Read the model definition and answer for the solid it produces. Units are mm, in the model's axes. A direction names the side the tool comes from. Coordinates: 2 decimals unless noted, no trailing zeros. Order: outer loops, then holes, each group sorted by start corner. A loop starts at its lowest first (then second) coordinate and runs counter-clockwise, first axis right, second up. Notation, with made-up numbers: (-27, -20) -> (2, -20) arc R20 cw to (2, -13) -> close; hole circle Ø10 at (40.25, 68). An arc over 180 degrees is marked (long way). Use CSV: the item, a comma, the result in double quotes.
```python
from build123d import *

# Parameters (mm, degrees)
BOSS_EXTRUDE1_DEPTH = 20.9804
CUT_EXTRUDE1_DEPTH  = 15.9004


with BuildPart() as part:
    # Sketch1 → Boss-Extrude1 (new body)
    with BuildSketch(Plane(origin=(0, 0, 0), x_dir=(1, 0, 0), z_dir=(0, 1, 0))):
        with BuildLine():
            Line((0, -8.255), (0, -23.876))
            ThreePointArc((0, -23.876), (0.92993597, -26.12106403), (3.175, -27.051))
            Line((3.175, -27.051), (16.330087154, -27.051))
            ThreePointArc((16.330087154, -27.051), (18.092140644, -27.584827438), (19.261669723, -29.0068))
            ThreePointArc((19.261669723, -29.0068), (30.988, -36.83), (42.714330277, -29.0068))
            ThreePointArc((42.714330277, -29.0068), (43.883859356, -27.584827438), (45.645912846, -27.051))
            Line((45.645912846, -27.051), (58.801, -27.051))
            ThreePointArc((58.801, -27.051), (61.04606403, -26.12106403), (61.976, -23.876))
            Line((61.976, -23.876), (61.976, -8.255))
            ThreePointArc((61.976, -8.255), (58.256256121, 0.725256121), (49.276, 4.445))
            Line((49.276, 4.445), (12.7, 4.445))
            ThreePointArc((12.7, 4.445), (3.719743879, 0.725256121), (0, -8.255))
        make_face()
        with BuildLine():
            Line((13.208, -10.541), (22.733, -10.541))
            ThreePointArc((22.733, -10.541), (25.908, -13.716), (22.733, -16.891))
            Line((22.733, -16.891), (13.208, -16.891))
            ThreePointArc((13.208, -16.891), (10.033, -13.716), (13.208, -10.541))
        make_face(mode=Mode.SUBTRACT)
        with BuildLine():
            Line((48.768, -10.541), (39.243, -10.541))
            ThreePointArc((39.243, -10.541), (36.068, -13.716), (39.243, -16.891))
            Line((39.243, -16.891), (48.768, -16.891))
            ThreePointArc((48.768, -16.891), (51.943, -13.716), (48.768, -10.541))
        make_face(mode=Mode.SUBTRACT)
    extrude(amount=BOSS_EXTRUDE1_DEPTH)

    # Sketch2 → Cut-Extrude1 (cut)
    with BuildSketch(Plane(origin=(0, 20.9804, 0), x_dir=(1, 0, 0), z_dir=(0, 1, 0))):
        with BuildLine():
            Line((6.858, -9.525), (6.858, -17.907))
            ThreePointArc((6.858, -17.907), (7.78793597, -20.15206403), (10.033, -21.082))
            Line((10.033, -21.082), (25.908, -21.082))
            ThreePointArc((25.908, -21.082), (28.15306403, -20.15206403), (29.083, -17.907))
            Line((29.083, -17.907), (29.083, -9.525))
            ThreePointArc((29.083, -9.525), (28.15306403, -7.27993597), (25.908, -6.35))
            Line((25.908, -6.35), (10.033, -6.35))
            ThreePointArc((10.033, -6.35), (7.78793597, -7.27993597), (6.858, -9.525))
        make_face()
        with BuildLine():
            Line((51.943, -6.35), (36.068, -6.35))
            ThreePointArc((36.068, -6.35), (33.82293597, -7.27993597), (32.893, -9.525))
            Line((32.893, -9.525), (32.893, -17.907))
            ThreePointArc((32.893, -17.907), (33.82293597, -20.15206403), (36.068, -21.082))
            Line((36.068, -21.082), (51.943, -21.082))
            ThreePointArc((51.943, -21.082), (54.18806403, -20.15206403), (55.118, -17.907))
            Line((55.118, -17.907), (55.118, -9.525))
            ThreePointArc((55.118, -9.525), (54.18806403, -7.27993597), (51.943, -6.35))
        make_face()
    extrude(amount=-CUT_EXTRUDE1_DEPTH, mode=Mode.SUBTRACT)


solid = part.part
```
Item 1: A tool of negligible diameter and unlimited length cuts with its end or side. For faces 1 (the cylindrical face through (33.8, 13.14, 20.13)), 2 (the flat face through (44, 3, 10.541)), 3 (the flat face through (52, 10, 27.051)), from which of +Z, -Z, +X, -X, +Y, -Y can it reach the whole face along a straight path? Write none if from no direction.
Return value:
face 1,"+Y"
face 2,"+Y, -Y"
face 3,"+Z, +X, +Y, -Y"
Item 2: Find section D-D, the plane y = 4. Give the vertices of the cut face in (x, z) (3 decimals), then the cut area to 3 significant figures.
Return value:
outline,"(0, 8.255) arc R12.7 ccw to (12.7, -4.445) -> (49.276, -4.445) arc R12.7 ccw to (61.976, 8.255) -> (61.976, 23.876) arc R3.175 ccw to (58.801, 27.051) -> (45.646, 27.051) arc R3.175 cw to (42.714, 29.007) arc R12.7 ccw to (19.262, 29.007) arc R3.175 cw to (16.33, 27.051) -> (3.175, 27.051) arc R3.175 ccw to (0, 23.876) -> close; hole (13.208, 10.541) -> (22.733, 10.541) arc R3.175 ccw to (22.733, 16.891) -> (13.208, 16.891) arc R3.175 ccw to start; hole (39.243, 10.541) -> (48.768, 10.541) arc R3.175 ccw to (48.768, 16.891) -> (39.243, 16.891) arc R3.175 ccw to start"
area,"1,880 mm^2"
Item 3: Find section B-B, the plane z = 15. Give the vertices of the cut face in (x, y), then the cut area to 3 significant figures.
Return value:
outline,"(0, 0) -> (10.3, 0) -> (10.3, 5.08) -> (6.86, 5.08) -> (6.86, 20.98) -> (0, 20.98) -> close; (25.64, 0) -> (36.34, 0) -> (36.34, 5.08) -> (32.89, 5.08) -> (32.89, 20.98) -> (29.08, 20.98) -> (29.08, 5.08) -> (25.64, 5.08) -> close; (51.67, 0) -> (61.98, 0) -> (61.98, 20.98) -> (55.12, 20.98) -> (55.12, 5.08) -> (51.67, 5.08) -> close"
area,"438 mm^2"
Item 4: Find section A-A, the plane y = 7.5. Give the vertices of the cut face in (x, z) (3 decimals), then the cut area to 3 significant figures.
Return value:
outline,"(0, 8.255) arc R12.7 ccw to (12.7, -4.445) -> (49.276, -4.445) arc R12.7 ccw to (61.976, 8.255) -> (61.976, 23.876) arc R3.175 ccw to (58.801, 27.051) -> (45.646, 27.051) arc R3.175 cw to (42.714, 29.007) arc R12.7 ccw to (19.262, 29.007) arc R3.175 cw to (16.33, 27.051) -> (3.175, 27.051) arc R3.175 ccw to (0, 23.876) -> close; hole (6.858, 9.525) arc R3.175 ccw to (10.033, 6.35) -> (25.908, 6.35) arc R3.175 ccw to (29.083, 9.525) -> (29.083, 17.907) arc R3.175 ccw to (25.908, 21.082) -> (10.033, 21.082) arc R3.175 ccw to (6.858, 17.907) -> close; hole (32.893, 9.525) arc R3.175 ccw to (36.068, 6.35) -> (51.943, 6.35) arc R3.175 ccw to (55.118, 9.525) -> (55.118, 17.907) arc R3.175 ccw to (51.943, 21.082) -> (36.068, 21.082) arc R3.175 ccw to (32.893, 17.907) -> close"
area,"1,420 mm^2"
Item 5: Each of these flat-tipped pins is pushed along its axis until it touches: P1, Ø10, axis at x = 17.5, z = 17, coming from the +Y side; P2, Ø6, axis at y = 14, z = 31.5, coming from the -X side; P3, Ø1.5, axis at y = 7, z = 3.5, coming from the +X side; P4, Ø12, axis at x = 45.5, z = 12.5, coming from the +Y side. Where does it stop, or does it pass through?
Return value:
P1,"stops at y = 20.98"
P2,"stops at x = 18.99"
P3,"stops at x = 61.33"
P4,"stops at y = 5.08"
Item 6: Straight lines are drawn through the part: line 1 along X through (y, z) = (13.25, 11.5); line 2 along X through (y, z) = (14.25, 7.5); line 3 along Z through (x, y) = (16, 12.25) (3 decimals). For each, find the intervals that lie inside material, in ascending order.
Return value:
line 1,"x = 0 to 6.86, 29.08 to 32.89, 55.12 to 61.98"
line 2,"x = 0.02 to 7.59, 28.35 to 33.62, 54.39 to 61.95"
line 3,"z = -4.445 to 6.35, 21.082 to 27.051"
Item 7: Find section C-C, the plane x = 25. Give the vertices of the cut face in (y, z) (3 decimals).
Return value:
outline,"(0, -4.445) -> (20.98, -4.445) -> (20.98, 6.35) -> (5.08, 6.35) -> (5.08, 11.493) -> (0, 11.493) -> close; (0, 15.939) -> (5.08, 15.939) -> (5.08, 21.082) -> (20.98, 21.082) -> (20.98, 35.33) -> (0, 35.33) -> close"
Item 8: The mould has two halves that part along X. Classify faces 4 (the flat face through (55.118, 13, 14)), 5 (the flat face through (31, 20.98, 11)), 6 (the cylindrical face through (0.91, 10.34, 26.1)): +X half, -X half, draft (parallel to the pull), parting line (faces both ways), or undercut.
Return value:
face 4,"undercut"
face 5,"draft"
face 6,"-X half"
